Verification items for this drawing (mm, ordinates from the low corner). A direction names the side the tool comes from. Coordinates: 2 decimals unless noted, no trailing zeros. Write each loop counter-clockwise with the first axis right and the second up, starting at its lowest first coordinate (ties: lowest second). Pieces come first, ordered by that corner, then holes. Notation, with made-up numbers: M 38,11.25 L 79,11.25 A10 cw 79,19.25 Z; hole C -2.5,-28 d9. An arc over 180 degrees is marked long. Write each question's results on one line, items separated by ' | '.
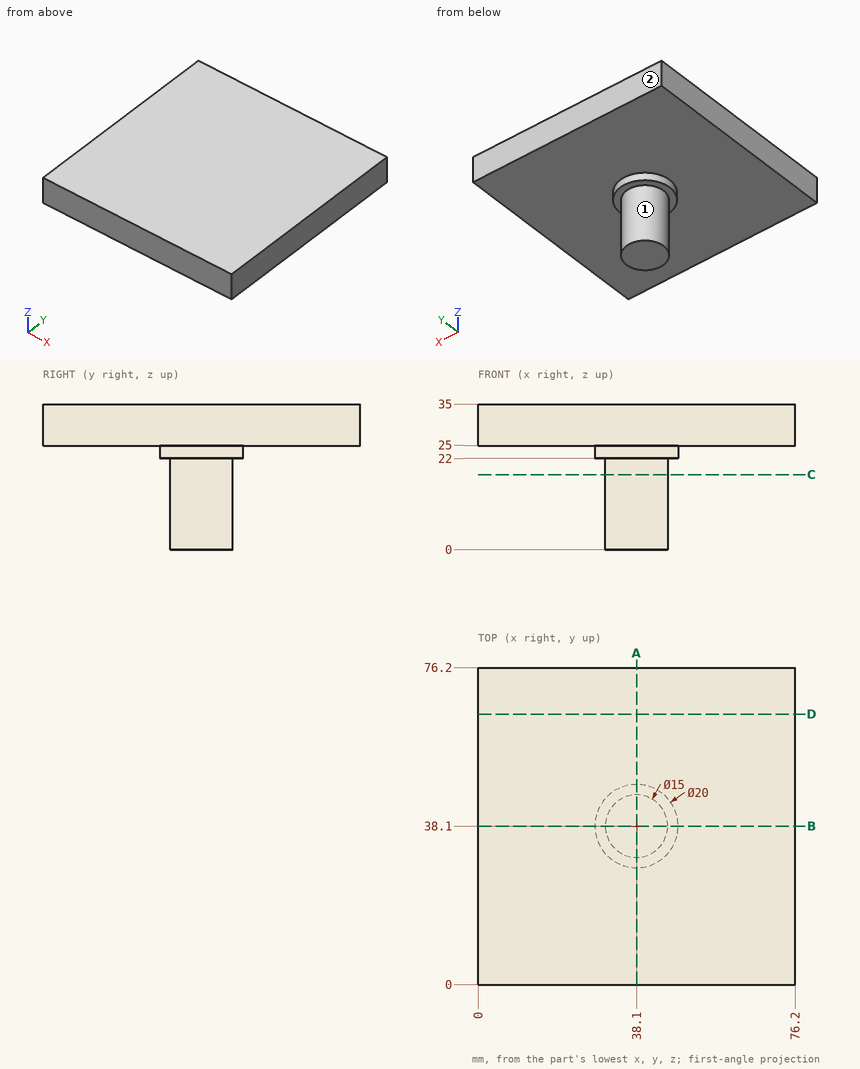
Q1. Access from +Z, -Z, +X, -X, +Y, -Y to the whole of each face (thin tool, end or side, straight path). Record for the marked faces 1 and 2.
Geometry check:
face 1: -Z | face 2: +Z, -Z, +X, -X, +Y
Q2. Scan lines: probe 1 along Z at (x, y) = (67, 53); probe 2 along X at (y, z) = (42, 7.5); probe 3 along X at (y, z) = (43.5, 21). Record each from-to range of solid material in increasing order.
Geometry check:
probe 1: z = 25 to 35 | probe 2: x = 31.69 to 44.51 | probe 3: x = 32.9 to 43.3
Q3. Sectioned sample at A-A on x = 38.1. Record the cut outline in (y, z).
Geometry check:
outline: M 0,25 L 28.1,25 L 28.1,22 L 30.6,22 L 30.6,0 L 45.6,0 L 45.6,22 L 48.1,22 L 48.1,25 L 76.2,25 L 76.2,35 L 0,35 Z
Q4. Depth check by flat-ended pin: P1, Ø12, axis at x = 56, z = 9, coming from the -Y side; P2, Ø10, axis at x = 15, y = 53.5, coming from the -Z side; P3, Ø16, axis at x = 40, y = 33.5, coming from the -Z side; P4, Ø10, axis at x = 48, z = 6, coming from the -Y side. Enter the tip coordinate at first touch or a pass-through.
Geometry check:
P1: passes through | P2: stops at z = 25 | P3: stops at z = 0 | P4: stops at y = 32.42
Q5. Sectioned sample at D-D on y = 65. Record the cut outline in (x, z), and give its area (3 significant figures).
Geometry check:
outline: M 0,25 L 76.2,25 L 76.2,35 L 0,35 Z | area: 762 mm2
Q6. Sectioned sample at C-C on z = 18. Record the cut outline in (x, y).
Geometry check:
outline: C 38.1,38.1 d15
